Autodesk Inventor part; units mm, degrees
ref_plane "YZ Plane" through (0, 0, 0) normal (1, 0, 0) x (0, 1, 0)
ref_plane "XZ Plane" through (0, 0, 0) normal (0, 1, 0) x (-1, 0, 0)
ref_plane "XY Plane" through (0, 0, 0) normal (0, 0, 1) x (1, 0, 0)
sketch "Boceto1" plane through (0, 0, 0) normal (0, 1, 0) x (-1, 0, 0)
  line L0 (0, 0) -> (100, 0)
  line L1 (100, 0) -> (100, -15)
  line L2 (100, -15) -> (0, -15)
  line L3 (0, -15) -> (0, 0)
  dimension "d0" = 100
  dimension "d1" = 15
extrude "Extrusión1" add sketch "Boceto1" along normal blind 10
sketch "Boceto3" plane through (0, 0, 0) normal (1, 0, 0) x (0, 0, -1)
  point P0 (0, 0)
chamfer "Chaflán1" distance 20 distance2 10 1 edges at (0, 10, -7.5) measured on face at (-33.3333, 10, -5)
sketch "Boceto4" plane through (0, 0, 0) normal (0, -1, 0) x (1, 0, 0)
  line L0 (0, -15) -> (-100, -15)
  line L1 (0, -15) -> (-100, -15)
  line L2 (-100, -15) -> (-100, 0)
  line L3 (-100, 0) -> (0, 0)
  line L4 (0, 0) -> (0, -15)
  dimension "d25" = 100
extrude "Extrusión2" add sketch "Boceto4" along normal blind 2
sketch "Boceto6" plane through (0, 10, 0) normal (0, 1, 0) x (1, 0, 0)
  line L0 (-100, 15) -> (-100, 0)
  line L1 (-100, 0) -> (-20, 0)
  point P0 (0, 0)
  point P1 (-92.5, 7.5)
  dimension "d26" = 7.5
  dimension "d27" = 7.5
hole "Agujero3" at (-92.5, 10, -7.5) direction (0, -1, 0) diameter 5.2 end through all counterbore diameter 11.7 counterbore depth 4
properties part number "cuña 10cm"
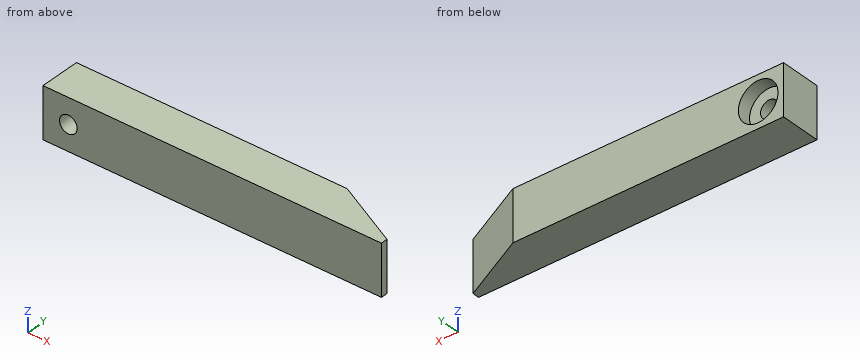
Source: CAD feature listing. Evaluate the final solid. Frame: model axes, mm. Give positions to 0.01 mm unless a question says otherwise; leave off trailing zeros. Write each loop counter-clockwise with the first axis right and the second up, starting at its lowest first coordinate (ties: lowest second). Pieces come first, ordered by that corner, then holes.
1. Section query D-D (z = -11.75). Return the cut outline in (x, y), then the cut area to 3 significant figures.
2. Section query A-A (z = -7.5). Return the cut outline in (x, y).
3. Section query B-B (x = -92.5). Return the cut outline in (y, z).
4. Section query C-C (y = 2). Return the cut outline in (x, z).
5. Material intervals for line 1 along Z through (x, y) = (-92.5, 7.5); line 2 along Z through (x, y) = (-92.5, 1.5); line 3 along X through (y, z) = (2, -7.5), sorted ascending.
6. First-contact query: pin 1 (2 mm diameter, centred on x = -85.5, y = 1, fed in from +Z). Flat tip, straight axial feed; report the tip coordinate or a pass-through.
Output values:
1. outline: (-100, -2) - (0, -2) - (0, 0) - (-20, 10) - (-88.48, 10) - (-88.48, 6) - (-96.52, 6) - (-96.52, 10) - (-100, 10) - close
1. area: 1,070 mm2
2. outline: (-100, -2) - (-95.1, -2) - (-95.1, 6) - (-98.35, 6) - (-98.35, 10) - (-100, 10) - close; (-89.9, -2) - (0, -2) - (0, 0) - (-20, 10) - (-86.65, 10) - (-86.65, 6) - (-89.9, 6) - close
3. outline: (-2, -15) - (10, -15) - (10, -13.35) - (6, -13.35) - (6, -10.1) - (-2, -10.1) - close; (-2, -4.9) - (6, -4.9) - (6, -1.65) - (10, -1.65) - (10, 0) - (-2, 0) - close
4. outline: (-100, -15) - (-4, -15) - (-4, 0) - (-100, 0) - close; hole circle Ø5.2 at (-92.5, -7.5)
5. line 1: z = -15 to -13.35, -1.65 to 0
5. line 2: z = -15 to -10.1, -4.9 to 0
5. line 3: x = -100 to -95.1, -89.9 to -4
6. pin 1: stops at z = 0
